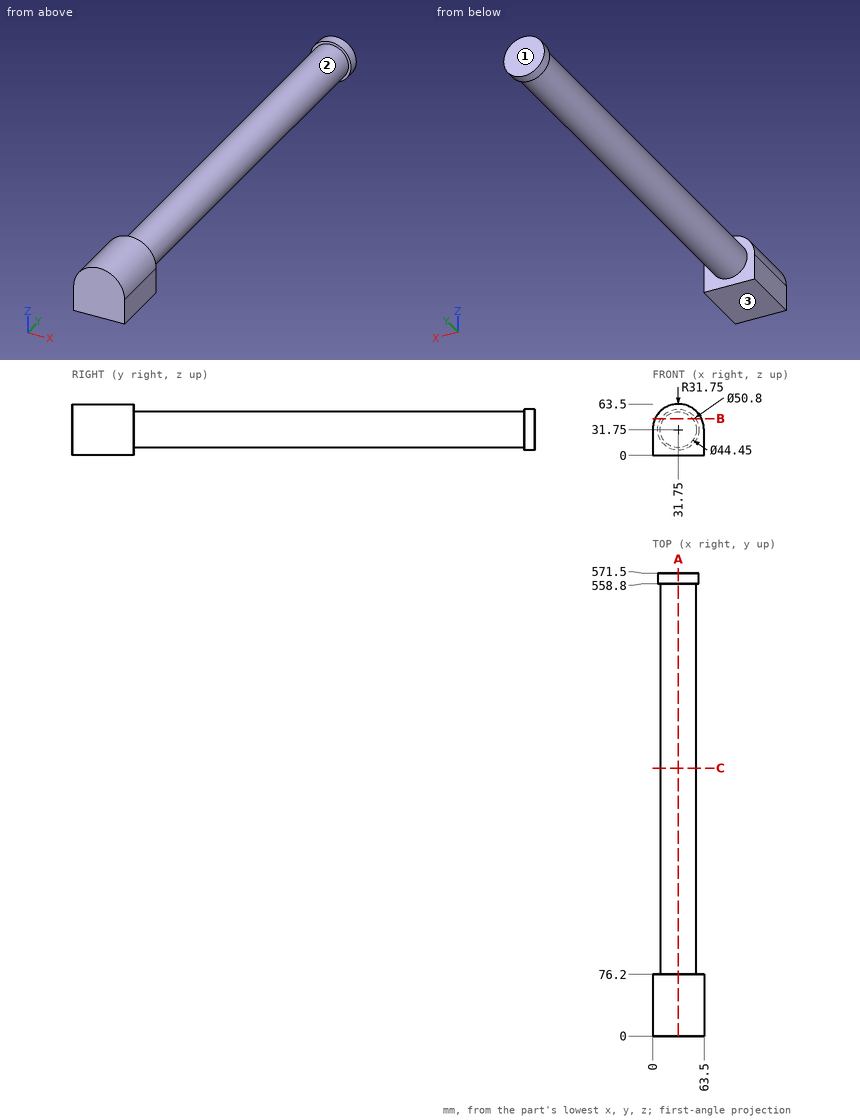
Print and shaded views of the part. All mm, measured from the part's lowest x, y and z. Round coordinates to 2 decimals unless told otherwise and drop trailing zeros. Write each loop counter-clockwise with the first axis right and the second up, starting at its lowest first coordinate (ties: lowest second). Pieces come first, ordered by that corner, then holes.
Item 1: Cut at A-A, the plane x = 31.75. Give the cut face in (y, z) (3 decimals).
Results:
outline: (0, 0) - (76.2, 0) - (76.2, 9.525) - (558.8, 9.525) - (558.8, 6.35) - (571.5, 6.35) - (571.5, 57.15) - (558.8, 57.15) - (558.8, 53.975) - (76.2, 53.975) - (76.2, 63.5) - (0, 63.5) - close
Item 2: Probe L1, parallel to Y at x = 23.5, z = 7.5; L2, parallel to X at y = 474.5, z = 14; L3, parallel to X at y = 118, z = 28.5. List the from-to ranges inside material, lowest first.
Results:
L1: y = 0 to 76.2
L2: x = 18.38 to 45.12
L3: x = 9.76 to 53.74
Item 3: Drop flat-ended pins along their axis: pin 1 Ø6 at (y, z) = (70.5, 57) entering from +X; pin 2 Ø5 at (y, z) = (502, 13.5) entering from -X; pin 3 Ø12 at (x, y) = (46, 378.5) entering from -Z. Give the stop position or say it passes through.
Results:
pin 1: stops at x = 54.4
pin 2: stops at x = 16.07
pin 3: stops at z = 11.11
Item 4: Two-plate mould, pull along Y, no slides. Class the marked faces 1, 2 and 3: +Y half, -Y half, draft (parallel to the pull), parting line (faces both ways), or undercut.
Results:
face 1: +Y half
face 2: undercut
face 3: draft
Item 5: Cut at C-C, the plane y = 331. Give the cut face in (x, z) (3 decimals), plus the area to 3 significant figures.
Results:
outline: circle Ø44.45 at (31.75, 31.75)
area: 1,550 mm2
Item 6: Cut at B-B, the plane z = 45.5. Give the cut face in (x, y).
Results:
outline: (3.13, 0) - (60.37, 0) - (60.37, 76.2) - (49.21, 76.2) - (49.21, 558.8) - (53.11, 558.8) - (53.11, 571.5) - (10.39, 571.5) - (10.39, 558.8) - (14.29, 558.8) - (14.29, 76.2) - (3.13, 76.2) - close
